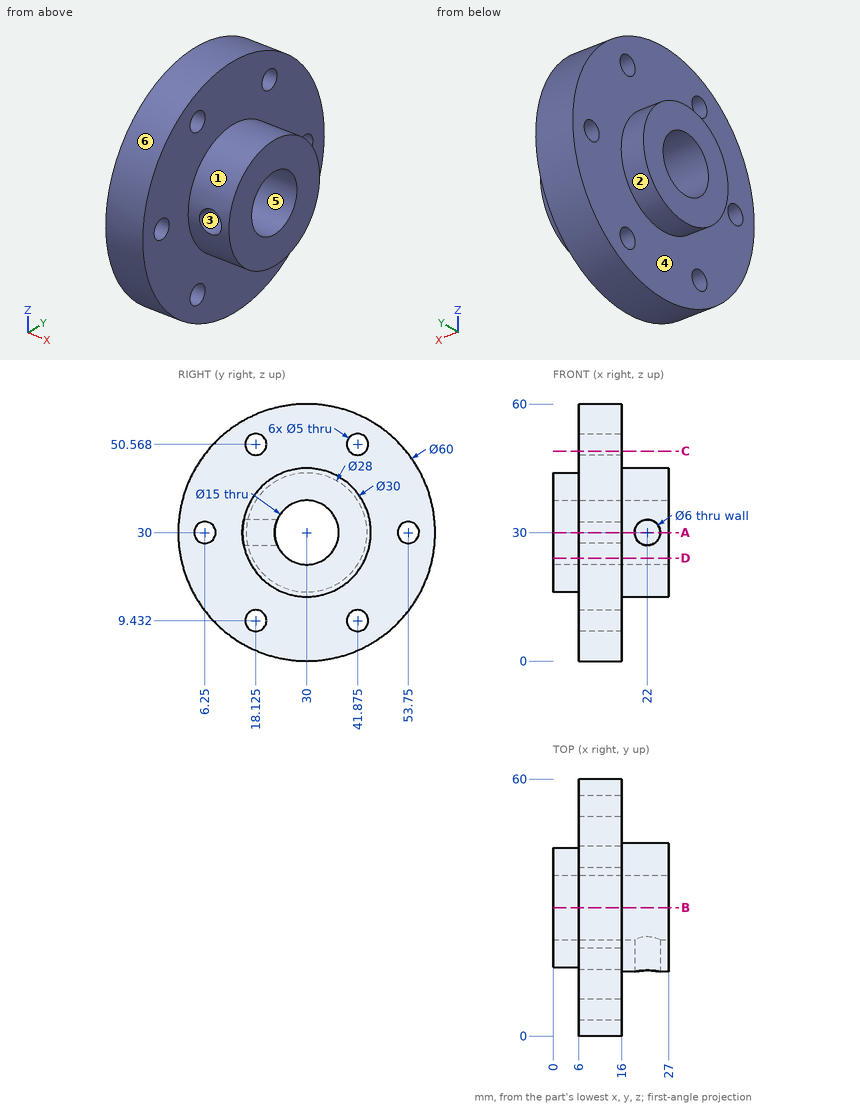
The figure shows three views and two pictorial views of one solid part (mm, origin at its lowest corner). Answer the questions. A direction names the side the tool comes from. Give positions to 0.01 mm unless a question says otherwise; leave off trailing zeros. Loops run counter-clockwise (first coordinate to the right, second up) from the corner with the lowest first, then second, coordinate; pieces in that order, holes last. Notation, with made-up numbers: (58.25, 19) -> (97.25, 19) arc R30 ccw to (97.25, 47) -> close; hole circle Ø10 at (71, 51.25). An arc over 180 degrees is marked (long way). Use CSV: the item, a comma, the result in double quotes.
1. The part is cut by section C-C (z = 49). Write down the section's boundary in (x, y), then the cut area to 3 significant figures.
Found:
outline,"(6, 6.78) -> (16, 6.78) -> (16, 16.18) -> (6, 16.18) -> close; (6, 20.07) -> (16, 20.07) -> (16, 39.93) -> (6, 39.93) -> close; (6, 43.82) -> (16, 43.82) -> (16, 53.22) -> (6, 53.22) -> close"
area,"386 mm^2"
2. A tool of negligible diameter and unlimited length cuts with its end or side. For the marked faces 1, 2 and 3, from which of +Z, -Z, +X, -X, +Y, -Y can it reach the whole face along a straight path? Write none if from no direction.
Found:
face 1,"+X"
face 2,"-X"
face 3,"-Y"
3. The part is cut by section D-D (z = 24). Write down the section's boundary in (x, y), then the cut area to 3 significant figures.
Found:
outline,"(0, 17.35) -> (6, 17.35) -> (6, 0.61) -> (16, 0.61) -> (16, 16.25) -> (27, 16.25) -> (27, 25.5) -> (0, 25.5) -> close; (0, 34.5) -> (27, 34.5) -> (27, 43.75) -> (16, 43.75) -> (16, 59.39) -> (6, 59.39) -> (6, 42.65) -> (0, 42.65) -> close"
area,"799 mm^2"
4. Straight lines are drawn through the part: line 1 (X direction, y = 17.5, z = 30); line 2 (Y direction, x = 16.5, z = 29.5); line 3 (X direction, y = 28, z = 53.5). For each, find the intervals that lie inside material, in ascending order.
Found:
line 1,"0 to 19, 25 to 27"
line 2,"15.01 to 22.52, 37.48 to 44.99"
line 3,"6 to 16"
5. Flat-ended cylindrical pins translate along their axes: pin 1 Ø2 at (x, y) = (12, 42) entering from -Z; pin 2 Ø5 at (x, z) = (21, 29.5) entering from +Y; pin 3 Ø5 at (x, z) = (22, 30) entering from -Y. Find the tip coordinate at first contact, or state that the pin passes through.
Found:
pin 1,"z = 2.09"
pin 2,"y = 45"
pin 3,"y = 37.07"
6. The part is cut by section B-B (y = 30). Write down the section's boundary in (x, z), then the cut area to 3 significant figures.
Found:
outline,"(0, 16) -> (6, 16) -> (6, 0) -> (16, 0) -> (16, 15) -> (27, 15) -> (27, 22.5) -> (0, 22.5) -> close; (0, 37.5) -> (27, 37.5) -> (27, 45) -> (16, 45) -> (16, 60) -> (6, 60) -> (6, 44) -> (0, 44) -> close"
area,"693 mm^2"
7. The mould has two halves that part along Y. Classify the marked faces 4, 5 and 6: +Y half, -Y half, draft (parallel to the pull), parting line (faces both ways), or undercut.
Found:
face 4,"draft"
face 5,"undercut"
face 6,"parting line"
8. The part is cut by section A-A (z = 30). Write down the section's boundary in (x, y).
Found:
outline,"(0, 16) -> (6, 16) -> (6, 8.75) -> (16, 8.75) -> (16, 15) -> (19, 15) -> (19, 22.5) -> (0, 22.5) -> close; (0, 37.5) -> (27, 37.5) -> (27, 45) -> (16, 45) -> (16, 51.25) -> (6, 51.25) -> (6, 44) -> (0, 44) -> close; (6, 0) -> (16, 0) -> (16, 3.75) -> (6, 3.75) -> close; (6, 56.25) -> (16, 56.25) -> (16, 60) -> (6, 60) -> close; (25, 15) -> (27, 15) -> (27, 22.5) -> (25, 22.5) -> close"
